from build123d import *

# Parameters (mm, degrees)
SKETCH1_W           = 120
SKETCH1_H           = 3
BOSS_EXTRUDE1_DEPTH = 220
SKETCH2_R           = 10
CUT_EXTRUDE1_DEPTH  = 10
SKETCH4_W           = 40
SKETCH4_H           = 40
CUT_EXTRUDE2_DEPTH  = 10


with BuildPart() as part:
    # Sketch1 → Boss-Extrude1 (new body)
    with BuildSketch(Plane.XY):
        with Locations((60, 1.5)):
            Rectangle(SKETCH1_W, SKETCH1_H)
    extrude(amount=BOSS_EXTRUDE1_DEPTH)

    # Sketch2 → Cut-Extrude1 (cut)
    with BuildSketch(Plane(origin=(0, 3, 0), x_dir=(1, 0, 0), z_dir=(0, 1, 0))):
        with Locations((60, -220)):
            Circle(SKETCH2_R)
        with Locations((60, 0)):
            Circle(SKETCH2_R)
    extrude(amount=-CUT_EXTRUDE1_DEPTH, mode=Mode.SUBTRACT)

    # Sketch4 → Cut-Extrude2 (cut)
    with BuildSketch(Plane(origin=(0, 3, 0), x_dir=(1, 0, 0), z_dir=(0, 1, 0))):
        with Locations((60, -60)):
            Rectangle(SKETCH4_W, SKETCH4_H)
    extrude(amount=-CUT_EXTRUDE2_DEPTH, mode=Mode.SUBTRACT)


solid = part.part
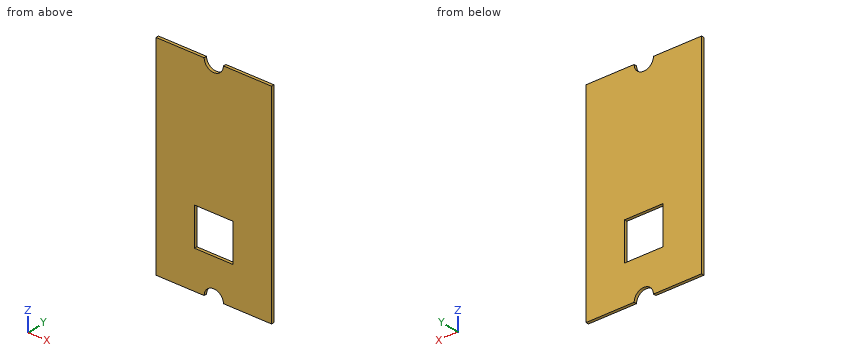
Verification items for the finished model (mm, model axes). Round coordinates to 2 decimals unless told otherwise and drop trailing zeros. Write each loop counter-clockwise with the first axis right and the second up, starting at its lowest first coordinate (ties: lowest second). Pieces come first, ordered by that corner, then holes.
(1) Section check C-C (z = 62.5). Enter the section's corners in (x, y), plus the area to 3 significant figures.
Returned:
outline: (0, 0) - (40, 0) - (40, 3) - (0, 3) - close; (80, 0) - (120, 0) - (120, 3) - (80, 3) - close
area: 240 mm2
(2) Section check A-A (x = 60). Enter the section's corners in (y, z).
Returned:
outline: (0, 10) - (3, 10) - (3, 40) - (0, 40) - close; (0, 80) - (3, 80) - (3, 210) - (0, 210) - close
(3) Section check B-B (y = 0.65). Enter the section's corners in (x, z).
Returned:
outline: (0, 0) - (50, 0) arc R10 cw to (70, 0) - (120, 0) - (120, 220) - (70, 220) arc R10 cw to (50, 220) - (0, 220) - close; hole (40, 40) - (80, 40) - (80, 80) - (40, 80) - close
(4) Depth check by flat-ended pin: pin 1 Ø8 at (x, z) = (29, 39.5) entering from -Y; pin 2 Ø1.5 at (x, y) = (59, 1.5) entering from +Z. Enter the tip coordinate at first touch or a pass-through.
Returned:
pin 1: stops at y = 0
pin 2: stops at z = 210.15
(5) Material ranges on line 1 (Z direction, x = 43, y = 2.2); line 2 (Z direction, x = 57, y = 0.25), recorded low to high.
Returned:
line 1: z = 0 to 40, 80 to 220
line 2: z = 9.54 to 40, 80 to 210.46
